Model file for the job. Use its own axes, mm. Face numbers are marked on the shaded views. A direction names the side the tool comes from. Round coordinates to 2 decimals unless told otherwise and drop trailing zeros. Loops run counter-clockwise (first coordinate to the right, second up) from the corner with the lowest first, then second, coordinate; pieces in that order, holes last. Notation, with made-up numbers: M 11,39.5 L 45,39.5 A32 cw 45,67.5 Z; hole C -39.75,-22 d8. An arc over 180 degrees is marked long. Use a Markdown table: item, result. Add a question column.
Q1. Probe line 1 (Y direction, x = 0.5, z = 0.1); line 2 (X direction, y = -0.7, z = -1.9) (3 decimals); line 3 (Z direction, x = -4.5, y = 2.05). List the from-to ranges inside material, lowest first. Write a range as from..to.
Q2. Tool access for the marked faces 1 and 2: list every direction of +Z, -Z, +X, -X, +Y, -Y with a clear straight run to the whole face (end or side of a thin tool).
Q3. Cut at A-A (x = 4.5). Give the cut face in (y, z).
Q4. Pin check, flat tips, straight feed: pin 1 (1 mm diameter, centred on y = 2, z = 1, fed in from +X); pin 2 (1.5 mm diameter, centred on x = -1.5, z = -1.5, fed in from +Y); pin 3 (1 mm diameter, centred on y = -2, z = -2, fed in from +X). Stop position of each tip, or through.
Q5. Cut at B-B (x = -1.25). Give the cut face in (y, z), plus the area to 3 significant figures.
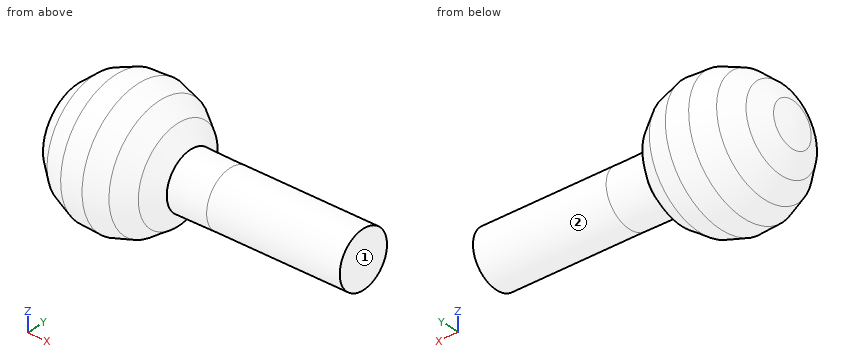
from build123d import *


with BuildPart() as part:
    # Ball_Stud Sketch → Ball_Stud (revolve)
    with BuildSketch(Plane.XY, mode=Mode.PRIVATE) as ball_stud_sk:
        Polygon((-7.5, 0), (-7.330102502, 0.995248625), (-6.839653449, 1.877770417), (-6.084203552, 2.547606545), (-5.149318842, 2.928888021), (-4.140889034, 2.978429001), (-3.173133929, 2.690618225), (-2.355666308, 2.098054579), (-1.781076639, 1.267854785), (0, 1.25), (6, 1.25), (6, 0), align=None)
    revolve(ball_stud_sk.sketch.rotate(Axis((-1000, 0, 0), (1, 0, 0)), 90), axis=Axis((-1000, 0, 0), (1, 0, 0)))


solid = part.part
Checked values:
| question | item | result |
|---|---|---|
| 1 | line 1 | y = -1.25..1.25 |
| 1 | line 2 | x = -6.674..-2.305 |
| 1 | line 3 | z = -2.14..2.14 |
| 2 | face 1 | +Z, -Z, +X, +Y, -Y |
| 2 | face 2 | +X |
| 3 | outline | C 0,0 d2.5 |
| 4 | pin 1 | stops at x = -2.11 |
| 4 | pin 2 | stops at y = 1.41 |
| 4 | pin 3 | stops at x = -2.67 |
| 5 | outline | C 0,0 d2.53 |
| 5 | area | 5.01 mm^2 |
